Study the drawing (mm; zero at the part's minimum x, y, z) and answer. Round coordinates to 2 decimals unless told otherwise and drop trailing zeros. Loops run counter-clockwise (first coordinate to the right, second up) from the corner with the lowest first, then second, coordinate; pieces in that order, holes last. Notation, with made-up numbers: (71, -19.75) - (94, -19.75) arc R12 ccw to (94, 0.25) - close; hole circle Ø10 at (-19, -14.75). An arc over 180 degrees is marked (long way). One line per item, written item: value.
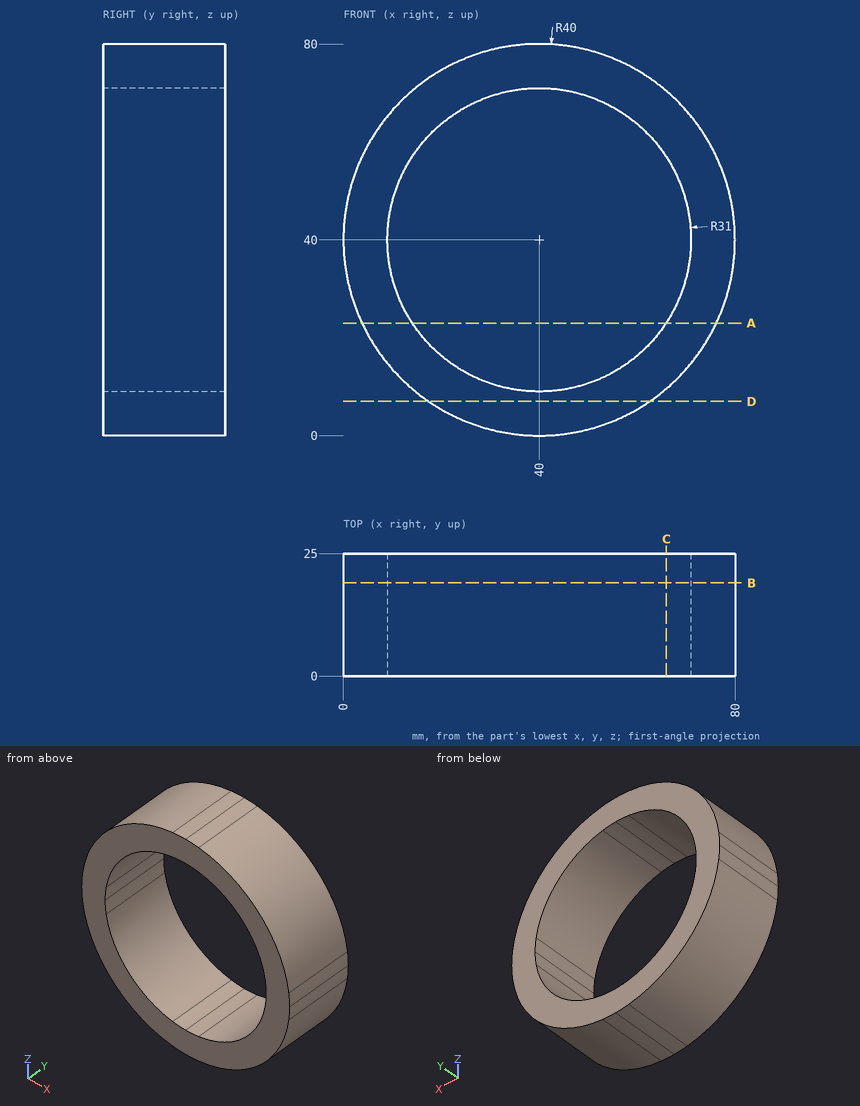
1) A cutting plane is placed at C-C on x = 66. Give the vertices of the cut face in (y, z), and give its area (3 significant figures).
Final values:
outline: (0, 9.6) - (25, 9.6) - (25, 23.12) - (0, 23.12) - close; (0, 56.88) - (25, 56.88) - (25, 70.4) - (0, 70.4) - close
area: 676 mm2
2) Each of these flat-tipped pins is pushed along its axis until it touches: pin 1 Ø6 at (y, z) = (17, 22.5) entering from +X; pin 2 Ø6 at (x, y) = (28.5, 7) entering from -Z; pin 3 Ø12 at (x, y) = (41.5, 19.5) entering from -Z; pin 4 Ø8 at (y, z) = (12.5, 10.5) entering from -X. Where does it stop, or does it pass through?
Final values:
pin 1: x = 77.28
pin 2: z = 0.91
pin 3: z = 0
pin 4: x = 9.18
3) A cutting plane is placed at B-B on y = 19. Give the vertices of the cut face in (x, z).
Final values:
outline: circle Ø80 at (40, 40); hole circle Ø62 at (40, 40)
4) A cutting plane is placed at D-D on z = 7. Give the vertices of the cut face in (x, y).
Final values:
outline: (17.39, 0) - (62.61, 0) - (62.61, 25) - (17.39, 25) - close
5) Consider L1, parallel to X at y = 15.5, z = 17.5; L2, parallel to Z at x = 56, y = 5.5; L3, parallel to X at y = 16, z = 27.5. Determine where each line is inside the solid, lowest interval first.
Final values:
L1: 6.93 to 18.68, 61.32 to 73.07
L2: 3.34 to 13.45, 66.55 to 76.66
L3: 2 to 11.63, 68.37 to 78
6) A cutting plane is placed at A-A on z = 23. Give the vertices of the cut face in (x, y), and give its area (3 significant figures).
Final values:
outline: (3.79, 0) - (14.08, 0) - (14.08, 25) - (3.79, 25) - close; (65.92, 0) - (76.21, 0) - (76.21, 25) - (65.92, 25) - close
area: 514 mm2
